Can you work these out from the model? Positions are in its coordinate system, mm. Face numbers are marked on the shaded views. A direction names the side the tool comes from. Round coordinates to 2 decimals unless told otherwise and drop trailing zeros. Loops run counter-clockwise (first coordinate to the right, second up) from the corner with the lowest first, then second, coordinate; pieces in that order, holes last.
from build123d import *

# Parameters (mm, degrees)
SKETCH1_R           = 40
BOSS_EXTRUDE1_DEPTH = 50
BOSS_EXTRUDE2_DEPTH = 15
SKETCH4_R           = 12.5
CUT_EXTRUDE1_DEPTH  = 35


with BuildPart() as part:
    # Sketch1 → Boss-Extrude1 (new body)
    with BuildSketch(Plane(origin=(0, 0, 0), x_dir=(1, 0, 0), z_dir=(0, 1, 0))):
        Circle(SKETCH1_R)
    extrude(amount=BOSS_EXTRUDE1_DEPTH)

    # Sketch2 → Boss-Extrude2 (add)
    with BuildSketch(Plane(origin=(0, 50, 0), x_dir=(1, 0, 0), z_dir=(0, 1, 0))):
        Polygon((0, -57.735026919), (50, -28.867513459), (50, 28.867513459), (0, 57.735026919), (-50, 28.867513459), (-50, -28.867513459), align=None)
    extrude(amount=BOSS_EXTRUDE2_DEPTH)

    # Sketch4 → Cut-Extrude1 (cut)
    with BuildSketch(Plane(origin=(0, 65, 0), x_dir=(1, 0, 0), z_dir=(0, 1, 0))):
        Circle(SKETCH4_R)
    extrude(amount=-CUT_EXTRUDE1_DEPTH, mode=Mode.SUBTRACT)


solid = part.part
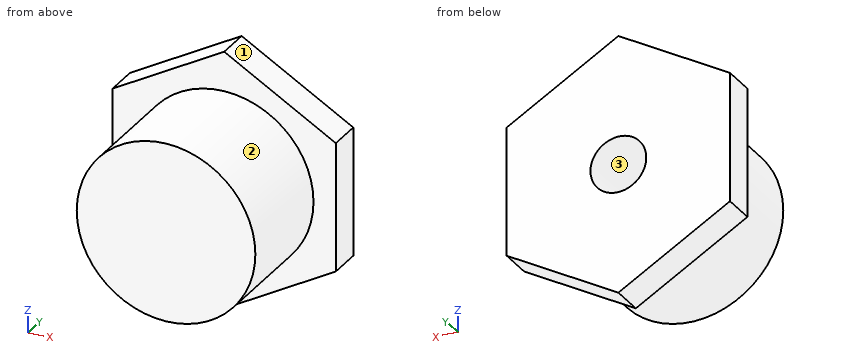
(1) For the marked faces 1, 2 and 3, which set-ups out of +Z, -Z, +X, -X, +Y, -Y let a thin tool reach every point of the face, with its end or its side?
Worked answers:
face 1: +Z, +X, +Y, -Y
face 2: -Y
face 3: +Y
(2) If we section it at B-B, the plane z = 0: List the corners of the cut face in (x, y) for me, then the cut area to 4 significant figures.
Worked answers:
outline: (-50, 50) - (-40, 50) - (-40, 0) - (40, 0) - (40, 50) - (50, 50) - (50, 65) - (12.5, 65) - (12.5, 30) - (-12.5, 30) - (-12.5, 65) - (-50, 65) - close
area: 4,625 mm2
(3) If I drill on line 1 (X direction, y = 40, z = 0); line 2 (X direction, y = 53.5, z = 0), over which ranges is the centre line in solid material (lowest first)?
Worked answers:
line 1: x = -40 to -12.5, 12.5 to 40
line 2: x = -50 to -12.5, 12.5 to 50
(4) If we section it at D-D, the plane y = 28: List the corners of the cut face in (x, z) for me, then the cut area to 3 significant figures.
Worked answers:
outline: circle Ø80 at (0, 0)
area: 5,030 mm2
(5) If we section it at C-C, the plane x = -28: List the corners of the cut face in (y, z) for me, then the cut area to 3 significant figures.
Worked answers:
outline: (0, -28.57) - (50, -28.57) - (50, -41.57) - (65, -41.57) - (65, 41.57) - (50, 41.57) - (50, 28.57) - (0, 28.57) - close
area: 4,100 mm2
(6) If we section it at A-A, the plane y = 57: List the corners of the cut face in (x, z) for me.
Worked answers:
outline: (-50, -28.87) - (0, -57.74) - (50, -28.87) - (50, 28.87) - (0, 57.74) - (-50, 28.87) - close; hole circle Ø25 at (0, 0)
(7) Will these pins go through, and if not, where does the flat tip stop? P1, Ø6, axis at x = -2.5, z = 10.5, coming from the +Y side; P2, Ø1, axis at x = 14, y = 33, coming from the +Z side; P3, Ø22.5, axis at x = 0, z = 0, coming from the +Y side; P4, Ø10, axis at x = 18.5, y = 31, coming from the -Z side.
Worked answers:
P1: stops at y = 65
P2: stops at z = 37.65
P3: stops at y = 30
P4: stops at z = -37.65
